Read the model definition and answer for the solid it produces. Units are mm, in the model's axes. A direction names the side the tool comes from. Round coordinates to 2 decimals unless told otherwise and drop trailing zeros. Order: outer loops, then holes, each group sorted by start corner. A loop starts at its lowest first (then second) coordinate and runs counter-clockwise, first axis right, second up. Notation, with made-up numbers: (44, 15.25) -> (54, 15.25) arc R21 cw to (54, 40.25) -> close; hole circle Ø3 at (-14.75, -31). An arc over 180 degrees is marked (long way). One line per item, written item: value. Start each with the question number.
1. Section A-A (x = 32.5) is taken. Give the vertices of the cut face in (y, z).
2. Flat-ended cylindrical pins translate along their axes: pin 1 Ø5.5 at (y, z) = (-7, 7) entering from -X; pin 2 Ø11 at (x, y) = (5.5, -18.5) entering from +Z; pin 3 Ø16 at (y, z) = (8.5, 4.5) entering from +X. Find the tip coordinate at first contact, or state that the pin passes through.
3. Section B-B (y = -19) is taken. Give the vertices of the cut face in (x, z), then the cut area to 3 significant figures.
4. Consider line 1 (Y direction, x = -6, z = 12.25) (3 decimals); line 2 (Z direction, x = 9.5, y = -21.5); line 3 (X direction, y = 18.5, z = 0.25). Determine where each line is inside the solid, lowest interval first.
5. For faces 1 (the face through (3, -3.125, 12)), 2 (the face through (18, -10, 17)), 3 (the face through (3, 3.125, 12)), determine the directions among +Z, -Z, +X, -X, +Y, -Y from which every point of the face is accessible in a straight line to the end or side of a thin tool.
6. The mould has two halves that part along X. Classify faces 4 (the face through (0, 0, -3.75)), 5 (the face through (8.75, 7, 7)), 6 (the face through (15.537, -24.248, 0.053)), 7 (the face through (18.03, -0.14, 15)): released by +X, released by -X, zero draft, split by the parting line, or undercut.
from build123d import *

# Parameters (mm, degrees)
F1_DEPTH = 25
F0_W     = 10
F0_H     = 7.5
F2_DEPTH = 10
F3_DEPTH = 3.125
F5_R     = 2.5


# Not quite as in the source:
# - a feature names something its author has since deleted; it is built from what else it names


with BuildPart() as f1:
    # F0 (on Front) → F1 (new body, symmetric)
    with BuildSketch(Plane.XZ):
        Polygon((16.25, -3.75), (16.25, 3.75), (8.75, 3.75), (-16.25, 3.75), (-16.25, -3.75), align=None)
    extrude(amount=F1_DEPTH, both=True)

    # F0 (on Front) → F2 (join, symmetric)
    with BuildSketch(Plane.XZ):
        with BuildLine():
            Line((8.75, 3.75), (16.25, 3.75))
            Line((16.25, 3.75), (16.25, 10.63))
            ThreePointArc((16.25, 10.63), (18.0805826176, 15.0494173824), (22.5, 16.88))
            Line((22.5, 16.88), (23.75, 16.88))
            Line((23.75, 16.88), (23.75, 24.38))
            Line((23.75, 24.38), (22.5, 24.38))
            add(Edge.make_bspline(
                [(22.0015189443, 24.3709612705), (22.1674265419, 24.3749356352), (22.3335889493, 24.3779529773), (22.5, 24.38)],
                knots=[43.5574597922, 43.5574597922, 43.5574597922, 43.5574597922, 43.8994236864, 43.8994236864, 43.8994236864, 43.8994236864], degree=3))
            ThreePointArc((22.0015189443, 24.3709612705), (12.6026110889, 20.1748516354), (8.75, 10.63))
            Line((8.75, 10.63), (8.75, 3.75))
        make_face()
        with Locations((28.75, 20.63)):
            Rectangle(F0_W, F0_H)
    extrude(amount=F2_DEPTH, both=True)

    # F0 (on Front) → F3 (join, symmetric)
    with BuildSketch(Plane.XZ):
        with BuildLine():
            Line((-16.25, 3.75), (8.75, 3.75))
            Line((8.75, 3.75), (8.75, 10.63))
            ThreePointArc((8.75, 10.63), (12.6026110889, 20.1748516354), (22.0015189443, 24.3709612705))
            add(Edge.make_bspline(
                [(-16.25, 3.75), (-16.1291590572, 7.8315246284), (0.86913148, 23.864728791), (22.0015189443, 24.3709612705)],
                knots=[0, 0, 0, 0, 43.5574597922, 43.5574597922, 43.5574597922, 43.5574597922], degree=3))
        make_face()
    extrude(amount=F3_DEPTH, both=True)

    # F0 (on Front) → F4 (revolve)
    with BuildSketch(Plane.XZ):
        Polygon((33.75, 24.38), (33.75, 16.88), (33.75, 15), (43.75, 15), (43.75, 26.25), (33.75, 26.25), align=None)
    revolve(axis=Axis((33.75, 0, 20.625), (0, 0, -1)))

    # F5
    f5_edges = [f1.edges().sort_by_distance(p)[0] for p in [
        (-16.25, -25, 0),
        (16.25, -25, 0),
        (-16.25, 25, 0),
        (16.25, 25, 0),
    ]]
    fillet(f5_edges, radius=F5_R)


solid = f1.part
Answer:
1. outline: (-10, 16.88) -> (-9.92, 16.88) -> (-9.92, 15) -> (9.92, 15) -> (9.92, 16.88) -> (10, 16.88) -> (10, 24.38) -> (9.92, 24.38) -> (9.92, 26.25) -> (-9.92, 26.25) -> (-9.92, 24.38) -> (-10, 24.38) -> close
2. pin 1: x = 8.75
2. pin 2: z = 3.75
2. pin 3: x = 16.54
3. outline: (-16.25, -3.75) -> (16.25, -3.75) -> (16.25, 3.75) -> (-16.25, 3.75) -> close
3. area: 244 mm^2
4. line 1: -3.125 to 3.125
4. line 2: -3.75 to 3.75
4. line 3: -16.25 to 16.25
5. face 1: +Z, -X, -Y
5. face 2: +Z, +X, -X, -Y
5. face 3: +Z, -X, +Y
6. face 4: zero draft
6. face 5: released by -X
6. face 6: released by +X
6. face 7: undercut
